Verification items for this drawing (mm, ordinates from the low corner). Give positions to 0.01 mm unless a question says otherwise; leave off trailing zeros. Order: outer loops, then holes, each group sorted by start corner. A loop starts at its lowest first (then second) coordinate and runs counter-clockwise, first axis right, second up.
(1) Gauge pin test, flat ends, axial feed: pin 1 (1.6 mm diameter, centred on x = 2, z = 32, fed in from -Y) (3 decimals); pin 2 (1.6 mm diameter, centred on x = 1, y = 65.5, fed in from -Z) (3 decimals); pin 3 (1.6 mm diameter, centred on x = 2, y = 45.5, fed in from -Z) (3 decimals). Record the tip position at first contact, or that the pin passes through.
(2) Sectioned sample at B-B on z = 49. Record the cut outline in (x, y) (3 decimals), plus the area to 3 significant figures.
(3) Sectioned sample at A-A on y = 17.5. Record the cut outline in (x, z) (3 decimals), plus the area to 3 significant figures.
(4) Sectioned sample at C-C on x = 2.6. Count the separate pieces of the cut face and the enclosed holes in it, plus the area to 3 significant figures.
(5) Scan lines: L1, parallel to Z at x = 2.1, y = 64.5 (3 decimals); L2, parallel to Y at x = 1.55, z = 22; L3, parallel to Y at x = 1.95, z = 50 (3 decimals). Record each from-to range of solid material in increasing order.
(6) Sectioned sample at D-D on y = 50. Record the cut outline in (x, z) (3 decimals), plus the area to 3 significant figures.
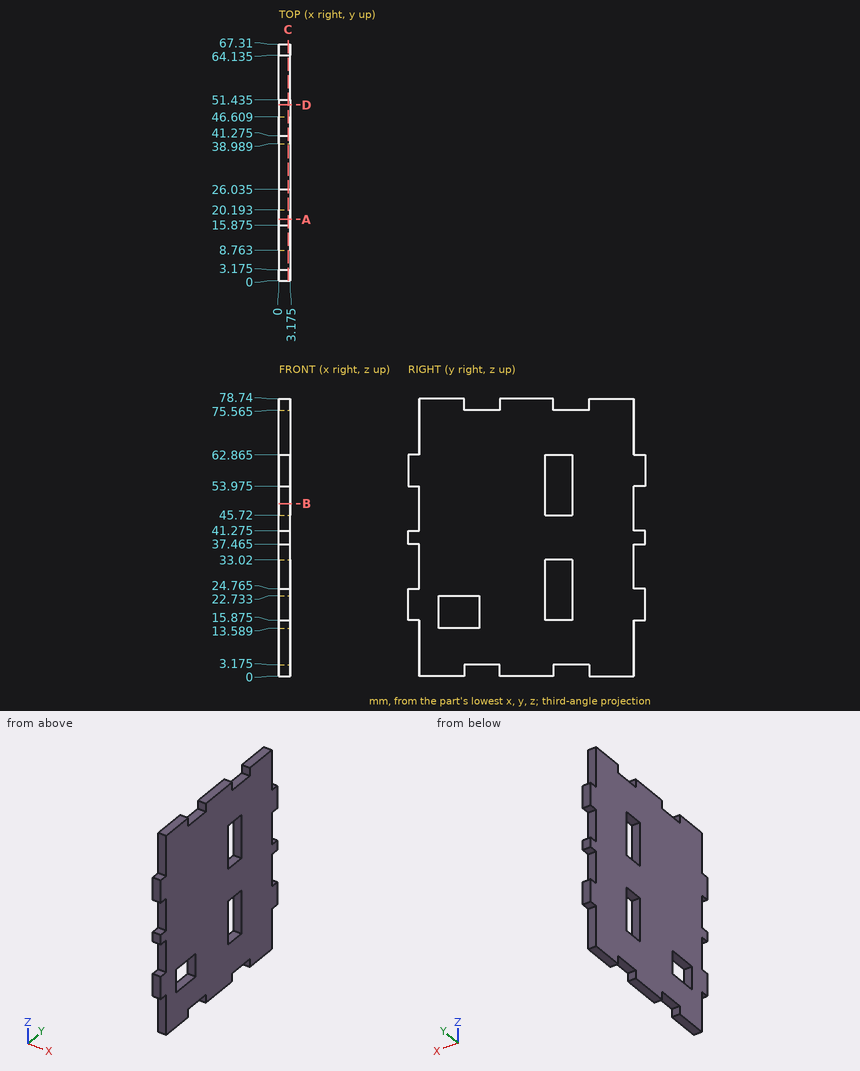
Ans:
1. pin 1: stops at y = 3.175
1. pin 2: stops at z = 15.875
1. pin 3: stops at z = 3.175
2. outline: (0, 3.175) - (3.175, 3.175) - (3.175, 38.989) - (0, 38.989) - close; (0, 46.609) - (3.175, 46.609) - (3.175, 64.135) - (0, 64.135) - close
2. area: 169 mm2
3. outline: (0, 3.175) - (3.175, 3.175) - (3.175, 13.589) - (0, 13.589) - close; (0, 22.733) - (3.175, 22.733) - (3.175, 75.565) - (0, 75.565) - close
3. area: 201 mm2
4. separate pieces: 1
4. enclosed holes: 3
4. area: 4,440 mm2
5. L1: z = 15.875 to 24.765, 37.465 to 41.275, 53.975 to 62.865
5. L2: y = 0 to 8.76, 20.19 to 38.99, 46.61 to 67.31
5. L3: y = 3.175 to 38.989, 46.609 to 64.135
6. outline: (0, 3.175) - (3.175, 3.175) - (3.175, 75.565) - (0, 75.565) - close
6. area: 230 mm2
